For this review, take the finished solid that the model builds, in its own axes (mm). A direction names the side the tool comes from. Coordinates: 2 decimals unless noted, no trailing zeros. Write each loop counter-clockwise with the first axis right and the second up, starting at its lowest first coordinate (ties: lowest second). Pieces come first, ordered by that corner, then holes. Notation, with made-up numbers: M 59.25,13 L 78.25,13 A29 cw 78.25,45 Z; hole C 66.5,-7.75 d7. An arc over 180 degrees is marked long. One line per question, with ' | ' between items.
from build123d import *

# Parameters (mm, degrees)
SKETCH1_W                      = 158
SKETCH1_H                      = 199.5
BOSS_EXTRUDE1_DEPTH            = 6.35
BOSS_EXTRUDE2_DEPTH            = 12.7
CBORE_FOR_M4_SHCS1_D           = 4.5
CBORE_FOR_M4_SHCS1_DEPTH       = 6.35
CBORE_FOR_M4_SHCS1_CBORE_D     = 8
CBORE_FOR_M4_SHCS1_CBORE_DEPTH = 4
FILLET2_R                      = 5
SKETCH11_W                     = 20
SKETCH11_H                     = 159
BOSS_EXTRUDE3_DEPTH            = 6.35
SKETCH12_R                     = 2.5
NUCLEO_DEPTH                   = 7.35
SKETCH13_R                     = 2.5
PIHOLDER_DEPTH                 = 7.35
SKETCH14_R                     = 2.5
ESTOP_DEPTH                    = 7.35
SKETCH15_R                     = 2.7
SKETCH15_R_2                   = 1.2
BUCKEXTRUDE_DEPTH              = 3
SKETCH16_R                     = 1.6
BUCKCUT_DEPTH                  = 7.35
LPATTERN1_COUNT                = 2
LPATTERN1_PITCH                = 28
SKETCH17_R                     = 1.6
IMU_DEPTH                      = 7.35
SKETCH19_R                     = 3.05
CUT_EXTRUDE8_DEPTH             = 3.1


with BuildPart() as part:
    # Sketch1 → Boss-Extrude1 (new body)
    with BuildSketch(Plane(origin=(0, 0, 0), x_dir=(1, 0, 0), z_dir=(0, 1, 0))):
        with Locations((79, -99.75)):
            Rectangle(SKETCH1_W, SKETCH1_H)
    extrude(amount=BOSS_EXTRUDE1_DEPTH)

    # Sketch3 → Boss-Extrude2 (add)
    with BuildSketch(Plane(origin=(0, 6.35, 0), x_dir=(1, 0, 0), z_dir=(0, 1, 0))):
        Polygon((0, 0), (0, -199.5), (158, -199.5), (158, -194.5), (5, -194.5), (5, 0), align=None)
    extrude(amount=BOSS_EXTRUDE2_DEPTH)

    # CBORE for M4 SHCS1
    with Locations(Plane(origin=(0, 6.35, 0), x_dir=(1, 0, 0), z_dir=(0, 1, 0))):
        with Locations((20, -55), (98, -179.5), (138, -179.5), (20, -130), (20, -105), (20, -30)):
            CounterBoreHole(CBORE_FOR_M4_SHCS1_D / 2, CBORE_FOR_M4_SHCS1_CBORE_D / 2, CBORE_FOR_M4_SHCS1_CBORE_DEPTH, depth=CBORE_FOR_M4_SHCS1_DEPTH)

    # Fillet2
    fillet2_edges = [part.edges().sort_by_distance(p)[0] for p in [
        (5, 12.7, 194.5),
        (0, 9.525, 199.5),
    ]]
    fillet(fillet2_edges, radius=FILLET2_R)

    # Sketch11 → Boss-Extrude3 (add)
    with BuildSketch(Plane(origin=(0, 6.35, 0), x_dir=(1, 0, 0), z_dir=(0, 1, 0))):
        with Locations((168, -79.5)):
            Rectangle(SKETCH11_W, SKETCH11_H)
    extrude(amount=-BOSS_EXTRUDE3_DEPTH)

    # Sketch12 → Nucleo (cut, through all)
    with BuildSketch(Plane(origin=(0, 6.35, 0), x_dir=(1, 0, 0), z_dir=(0, 1, 0))):
        with Locations((168.2, -21)):
            Circle(SKETCH12_R)
        with Locations((168.2, -86.1)):
            Circle(SKETCH12_R)
        with Locations((85, -86.1)):
            Circle(SKETCH12_R)
        with Locations((85, -21)):
            Circle(SKETCH12_R)
    extrude(amount=-NUCLEO_DEPTH, mode=Mode.SUBTRACT)

    # Sketch13 → PIHolder (cut, through all)
    with BuildSketch(Plane(origin=(0, 6.35, 0), x_dir=(1, 0, 0), z_dir=(0, 1, 0))):
        with Locations((59, -143)):
            Circle(SKETCH13_R)
        with Locations((10, -143)):
            Circle(SKETCH13_R)
        with Locations((10, -85)):
            Circle(SKETCH13_R)
        with Locations((59, -85)):
            Circle(SKETCH13_R)
    extrude(amount=-PIHOLDER_DEPTH, mode=Mode.SUBTRACT)

    # Sketch14 → ESTOP (cut, through all)
    with BuildSketch(Plane(origin=(0, 6.35, 0), x_dir=(1, 0, 0), z_dir=(0, 1, 0))):
        with Locations((170, -134.5)):
            Circle(SKETCH14_R)
        with Locations((142.875, -161.625)):
            Circle(SKETCH14_R)
    extrude(amount=-ESTOP_DEPTH, mode=Mode.SUBTRACT)

    # Sketch15 → BuckExtrude (add)
    with BuildSketch(Plane(origin=(0, 6.35, 0), x_dir=(1, 0, 0), z_dir=(0, 1, 0))):
        with Locations((116, -138.1)):
            Circle(SKETCH15_R)
        with Locations((116, -138.1)):
            Circle(SKETCH15_R_2, mode=Mode.SUBTRACT)
        with Locations((99, -168.9)):
            Circle(SKETCH15_R)
        with Locations((99, -168.9)):
            Circle(SKETCH15_R_2, mode=Mode.SUBTRACT)
    buckextrude = extrude(amount=BUCKEXTRUDE_DEPTH)

    # Sketch16 → BuckCut (cut, through all)
    with BuildSketch(Plane(origin=(0, 6.35, 0), x_dir=(1, 0, 0), z_dir=(0, 1, 0))):
        with Locations((99, -168.9)):
            Circle(SKETCH16_R)
        with Locations((116, -138.1)):
            Circle(SKETCH16_R)
    buckcut = extrude(amount=-BUCKCUT_DEPTH, mode=Mode.SUBTRACT)

    # LPattern1: BuckExtrude, BuckCut ×2
    with Locations(*[(-i * LPATTERN1_PITCH, 0, 0) for i in range(1, LPATTERN1_COUNT)]):
        add(buckextrude)
        add(buckcut, mode=Mode.SUBTRACT)

    # Sketch17 → IMU (cut, through all)
    with BuildSketch(Plane(origin=(0, 6.35, 0), x_dir=(1, 0, 0), z_dir=(0, 1, 0))):
        with Locations((28.89, -55.84)):
            Circle(SKETCH17_R)
        with Locations((28.89, -76.16)):
            Circle(SKETCH17_R)
        with Locations((11.11, -76.16)):
            Circle(SKETCH17_R)
        with Locations((11.11, -55.84)):
            Circle(SKETCH17_R)
    extrude(amount=-IMU_DEPTH, mode=Mode.SUBTRACT)

    # Sketch19 → Cut-Extrude8 (cut)
    with BuildSketch(Plane(origin=(0, 6.35, 0), x_dir=(1, 0, 0), z_dir=(0, 1, 0))):
        with Locations((126.6, -6)):
            Circle(SKETCH19_R)
        with Locations((85, -6)):
            Circle(SKETCH19_R)
        with Locations((116, -116.1)):
            Circle(SKETCH19_R)
        with Locations((71, -116.1)):
            Circle(SKETCH19_R)
        with Locations((71, -21)):
            Circle(SKETCH19_R)
        with Locations((71, -61)):
            Circle(SKETCH19_R)
        with Locations((41, -61)):
            Circle(SKETCH19_R)
        with Locations((41, -21)):
            Circle(SKETCH19_R)
    extrude(amount=-CUT_EXTRUDE8_DEPTH, mode=Mode.SUBTRACT)


solid = part.part
1) Machinability: for faces 5 (the flat face through (117, 9.35, 137)), 6 (the cylindrical face through (18.962, 1.159, 131.996)), 7 (the cylindrical face through (129.51, 4.82, 5.08)), which of the approach directions +Z, -Z, +X, -X, +Y, -Y give a long, thin tool a straight path to every point of the face, cutting with its end or side? Answer none if there is none.
Responses:
face 5: -Z, +X, +Y | face 6: +Y, -Y | face 7: +Y
2) We need section C-C on y = 11.75. State the section outline as (x, z) points, then the cut area to 3 significant figures.
Responses:
outline: M 0,0 L 5,0 L 5,189.5 A5 cw 10,194.5 L 158,194.5 L 158,199.5 L 5,199.5 A5 ccw 0,194.5 Z | area: 1,760 mm^2
3) To check wall thickness, follow line 1 along X through (y, z) = (2.75, 168.9); line 2 along X through (y, z) = (0.75, 179.5); line 3 along Z through (x, y) = (20, 3.5). State the ranges of each line that lie inside material, in increasing order. Write a range as [from, to].
Responses:
line 1: [0, 69.4], [72.6, 97.4], [100.6, 158] | line 2: [0, 95.75], [100.25, 135.75], [140.25, 158] | line 3: [0, 26], [34, 51], [59, 101], [109, 126], [134, 199.5]
4) We need section A-A on x = 59. State the section outline as (y, z) points.
Responses:
outline: M 0,0 L 6.35,0 L 6.35,82.5 L 0,82.5 Z; M 0,87.5 L 6.35,87.5 L 6.35,140.5 L 0,140.5 Z; M 0,145.5 L 6.35,145.5 L 6.35,194.5 L 19.05,194.5 L 19.05,199.5 L 0,199.5 Z
5) We need section B-B on z = 6. State the section outline as (x, y) points.
Responses:
outline: M 0,0 L 178,0 L 178,6.35 L 129.65,6.35 L 129.65,3.25 L 123.55,3.25 L 123.55,6.35 L 88.05,6.35 L 88.05,3.25 L 81.95,3.25 L 81.95,6.35 L 5,6.35 L 5,19.05 L 0,19.05 Z
6) Insertion check: pin 1 Ø1 at (x, z) = (19.5, 22) entering from -Y; pin 2 Ø4 at (y, z) = (11.5, 60.5) entering from +X; pin 3 Ø3 at (x, z) = (42, 20.5) entering from +Y; pin 4 Ø6.5 at (x, z) = (41, 61) entering from +Y. Each pin has a flat end and moves straight along its axis. Give the tip position at first contact, or say it passes through.
Responses:
pin 1: y = 0 | pin 2: x = 5 | pin 3: y = 3.25 | pin 4: y = 6.35
7) We need section D-D on x = 126.6. State the section outline as (y, z) points, then the cut area to 3 significant figures.
Responses:
outline: M 0,0 L 6.35,0 L 6.35,2.95 L 3.25,2.95 L 3.25,9.05 L 6.35,9.05 L 6.35,194.5 L 19.05,194.5 L 19.05,199.5 L 0,199.5 Z | area: 1,310 mm^2
8) The part is to be moulded in two halves that separate along Z. For faces 1 (the cylindrical face through (117.246, 7.829, 140.495)), 2 (the flat face through (140, 2.35, 181)), 3 (the flat face through (178, 3, 81)), 4 (the cylindrical face through (1.43, 9.66, 198)), say which applies: +Z half, -Z half, draft (parallel to the pull), parting line (faces both ways), or undercut.
Responses:
face 1: undercut | face 2: undercut | face 3: draft | face 4: +Z half
